Read the model definition and answer for the solid it produces. Units are mm, in the model's axes. A direction names the side the tool comes from. Round coordinates to 2 decimals unless told otherwise and drop trailing zeros. Write each loop counter-clockwise with the first axis right and the second up, starting at its lowest first coordinate (ties: lowest second). Pieces come first, ordered by that corner, then holes. Notation, with made-up numbers: (-27, 85.5) - (2, 85.5) arc R15 ccw to (2, 111.5) - close; hole circle Ø9 at (18, 72.25). An arc over 180 degrees is marked (long way). One line per item, written item: value. Start each with the question number.
(1) Find the intervals of material crossed by L1, parallel to X at y = 12, z = 7.25; L2, parallel to Z at x = 14.55, y = 1.1; L3, parallel to Y at x = 8, z = 8.25, in increasing order.
(2) A cutting plane is placed at B-B, the plane y = 11.75. Determine the outline of the cut face in (x, z), plus the area to 3 significant figures.
(3) Flat-ended cylindrical pins translate along their axes: pin 1 Ø4.5 at (x, z) = (-14.55, 4.25) entering from +Y; pin 2 Ø1.5 at (x, z) = (-0.5, 7.5) entering from -Y; pin 3 Ø4 at (y, z) = (8, 5) entering from +X. Find the tip coordinate at first contact, or state that the pin passes through.
(4) A cutting plane is placed at C-C, the plane z = 4.25. Determine the outline of the cut face in (x, y).
(5) For faces 1 (the face through (16, 1.5, 3)), 2 (the face through (9.8, 9, 4)), 3 (the face through (-11.3, 10, 4)), determine the directions among +Z, -Z, +X, -X, +Y, -Y from which every point of the face is accessible in a straight line to the end or side of a thin tool.
(6) The mould has two halves that part along X. Classify faces 4 (the face through (12.98, 0.76, 3.6)), 5 (the face through (17.8, 1, 4)), 6 (the face through (-16, 1.5, 3)), 7 (the face through (-11.601, 1.785, 4.31)): +X half, -X half, draft (parallel to the pull), parting line (faces both ways), or undercut.
(7) A cutting plane is placed at D-D, the plane x = -2. Determine the outline of the cut face in (y, z).
(8) A cutting plane is placed at A-A, the plane x = 14.55. Determine the outline of the cut face in (y, z), plus the area to 3 significant figures.
from build123d import *

# Parameters (mm, degrees)
BOSS_EXTRUDE1_DEPTH = 8.5
SKETCH2_R           = 1.7
CUT_EXTRUDE1_DEPTH  = 27.362664888
FILLET1_R           = 1


with BuildPart() as part:
    # Sketch1 → Boss-Extrude1 (new body)
    with BuildSketch(Plane.XY):
        Polygon((-17.8, 0), (-17.8, 1.5), (-11.3, 1.5), (-11.3, 18.99), (11.3, 18.99), (11.3, 1.5), (17.8, 1.5), (17.8, 0), (9.8, 0), (9.8, 17.49), (-9.8, 17.49), (-9.8, 0), align=None)
    extrude(amount=BOSS_EXTRUDE1_DEPTH)

    # Sketch2 → Cut-Extrude1 (cut, through all)
    with BuildSketch(Plane(origin=(0, 1.5, 0), x_dir=(1, 0, 0), z_dir=(0, 1, 0))):
        with Locations(Location((14.55, -4.25, 0), (0, 0, 180))):
            Circle(SKETCH2_R)
    cut_extrude1 = extrude(amount=-CUT_EXTRUDE1_DEPTH, mode=Mode.SUBTRACT)

    # Fillet1
    fillet1_edges = [part.edges().sort_by_distance(p)[0] for p in [
        (-11.3, 1.5, 4.25),
        (-11.3, 18.99, 4.25),
        (11.3, 18.99, 4.25),
        (11.3, 1.5, 4.25),
    ]]
    fillet(fillet1_edges, radius=FILLET1_R)

    # Mirror1: Cut-Extrude1 across plane
    add(cut_extrude1.mirror(Plane(origin=(0, 0, 0), x_dir=(0, 0, 1), z_dir=(1, 0, 0))), mode=Mode.SUBTRACT)


solid = part.part
Here are the results:
1. L1: -11.3 to -9.8, 9.8 to 11.3
1. L2: 0 to 2.55, 5.95 to 8.5
1. L3: 17.49 to 18.99
2. outline: (-11.3, 0) - (-9.8, 0) - (-9.8, 8.5) - (-11.3, 8.5) - close; (9.8, 0) - (11.3, 0) - (11.3, 8.5) - (9.8, 8.5) - close
2. area: 25.5 mm²
3. pin 1: y = 1.5
3. pin 2: y = 17.49
3. pin 3: x = 11.3
4. outline: (-17.8, 0) - (-16.25, 0) - (-16.25, 1.5) - (-17.8, 1.5) - close; (-12.85, 0) - (-9.8, 0) - (-9.8, 17.49) - (9.8, 17.49) - (9.8, 0) - (12.85, 0) - (12.85, 1.5) - (12.3, 1.5) arc R1 cw to (11.3, 2.5) - (11.3, 17.99) arc R1 ccw to (10.3, 18.99) - (-10.3, 18.99) arc R1 ccw to (-11.3, 17.99) - (-11.3, 2.5) arc R1 cw to (-12.3, 1.5) - (-12.85, 1.5) - close; (16.25, 0) - (17.8, 0) - (17.8, 1.5) - (16.25, 1.5) - close
5. face 1: +Z, -Z, +X, +Y
5. face 2: +Z, -Z, -Y
5. face 3: +Z, -Z, -X, +Y
6. face 4: undercut
6. face 5: +X half
6. face 6: draft
6. face 7: -X half
7. outline: (17.49, 0) - (18.99, 0) - (18.99, 8.5) - (17.49, 8.5) - close
8. outline: (0, 0) - (1.5, 0) - (1.5, 2.55) - (0, 2.55) - close; (0, 5.95) - (1.5, 5.95) - (1.5, 8.5) - (0, 8.5) - close
8. area: 7.65 mm²
